Source: CAD feature listing. Evaluate the final solid. Frame: model axes, mm. Face numbers are marked on the shaded views. A direction names the side the tool comes from. Give positions to 0.01 mm unless a question says otherwise; leave off trailing zeros. Order: outer loops, then holes, each group sorted by start corner. A loop starts at its lowest first (then second) coordinate and runs counter-clockwise, first axis right, second up. Notation, with made-up numbers: (43, 61.25) - (66, 61.25) arc R14 ccw to (66, 68.25) - close; hole circle Ø4 at (58, 52.5). An arc over 180 degrees is marked (long way). Write each question's results on one line, items separated by ' | '. Start each with the question number.
Item 1: Section D-D on x = 0. Output: boundary loops of the cut face in (y, z), and give its area (3 significant figures).
Item 2: Contact query for flat-ended pins moving along their axis: pin 1 Ø5 at (x, y) = (-1.5, 9) entering from +Z; pin 2 Ø10 at (x, z) = (9, 53.5) entering from -Y. Output: stop coordinate, or through.
Item 3: Section C-C on z = 38.5. Output: boundary loops of the cut face in (x, y).
Item 4: Line query: line 1 along X through (y, z) = (15.5, 23); line 2 along X through (y, z) = (-17, 12). Output: solid intervals per line, ascending.
Item 5: Set-up query: the marked faces 1 and 2. Return all of +Z, -Z, +X, -X, +Y, -Y with unobstructed straight access to the full face (end or side cutting, diameter ignored); none if empty.
Item 6: Section A-A on x = 15.5. Output: boundary loops of the cut face in (y, z).
```python
from build123d import *

# Parameters (mm, degrees)
F4_W     = 42.3
F4_H     = 42.3
F4_R     = 11
F5_DEPTH = 48
F4_R_2   = 2.5
F6_DEPTH = 50
F7_DEPTH = 74
F8_D     = 4.5
F8_DEPTH = 48
F8_TIP   = 1.3519363928


with BuildPart() as f5:
    # F4 (on Top) → F5 (new body)
    with BuildSketch(Plane.XY):
        Rectangle(F4_W, F4_H)
        Circle(F4_R, mode=Mode.SUBTRACT)
    extrude(amount=F5_DEPTH)

    # F4 (on Top) → F6 (join)
    with BuildSketch(Plane.XY):
        Circle(F4_R)
        Circle(F4_R_2, mode=Mode.SUBTRACT)
    extrude(amount=F6_DEPTH)

    # F4 (on Top) → F7 (join)
    with BuildSketch(Plane.XY):
        Circle(F4_R_2)
    extrude(amount=F7_DEPTH)

    # F8
    with Locations(Plane(origin=(0, 0, 0), x_dir=(1, 0, 0), z_dir=(0, 0, -1))):
        with Locations((15.5, -15.5), (-15.5, -15.5), (-15.5, 15.5), (15.5, 15.5)):
            Hole(F8_D / 2, depth=F8_DEPTH)
            with Locations((0, 0, -(F8_DEPTH + F8_TIP / 2))):  # 118° drill point
                Cone(0, F8_D / 2, F8_TIP, mode=Mode.SUBTRACT)


solid = f5.part
```
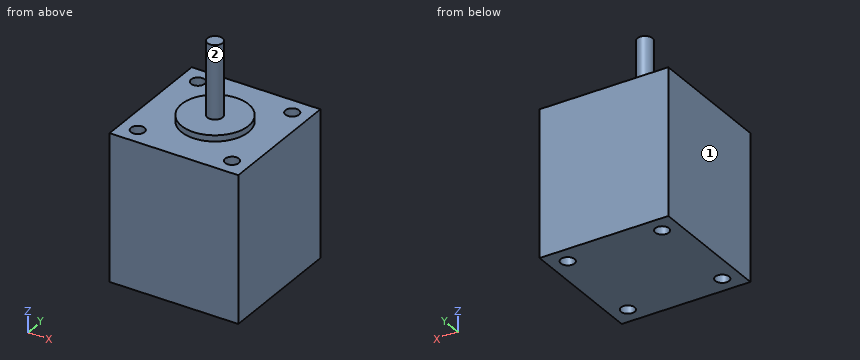
Evaluation:
1) outline: (-21.15, 0) - (21.15, 0) - (21.15, 48) - (11, 48) - (11, 50) - (2.5, 50) - (2.5, 74) - (-2.5, 74) - (-2.5, 50) - (-11, 50) - (-11, 48) - (-21.15, 48) - close | area: 2,190 mm^2
2) pin 1: stops at z = 50 | pin 2: stops at y = -9.57
3) outline: (-21.15, -21.15) - (21.15, -21.15) - (21.15, 21.15) - (-21.15, 21.15) - close; hole circle Ø4.5 at (-15.5, -15.5); hole circle Ø4.5 at (-15.5, 15.5); hole circle Ø4.5 at (15.5, -15.5); hole circle Ø4.5 at (15.5, 15.5)
4) line 1: x = -21.15 to -17.75, -13.25 to 13.25, 17.75 to 21.15 | line 2: x = -21.15 to -17.18, -13.82 to 13.82, 17.18 to 21.15
5) face 1: +Z, -Z, -X, +Y, -Y | face 2: +Z
6) outline: (-21.15, 0) - (-17.75, 0) - (-17.75, 48) - (-21.15, 48) - close; (-13.25, 0) - (13.25, 0) - (13.25, 48) - (-13.25, 48) - close; (17.75, 0) - (21.15, 0) - (21.15, 48) - (17.75, 48) - close
